Model file for the job. Use its own axes, mm. A direction names the side the tool comes from. Coordinates: 2 decimals unless noted, no trailing zeros. Loops run counter-clockwise (first coordinate to the right, second up) from the corner with the lowest first, then second, coordinate; pieces in that order, holes last.
from build123d import *

# Parameters (mm, degrees)
SZKIC1_R                    = 37.5
SZKIC1_R_2                  = 22.5
DODANIE_WYCI_GNI_CIE1_DEPTH = 41
SZKIC2_R                    = 35
SZKIC2_R_2                  = 25
WYTNIJ_WYCI_GNI_CIE1_DEPTH  = 1
SZKIC3_R                    = 5.05
SZKIC3_R_2                  = 37.5
DODANIE_WYCI_GNI_CIE2_DEPTH = 10
SZYK_KO_OWY1_OUTLINE_R      = 5.05
SZYK_KO_OWY1_DEPTH          = 10


# Read off the part's stored shape, not the designer's step: Szyk kołowy1
with BuildPart() as part:
    # Szkic1 → Dodanie-wyciągnięcie1 (new body)
    with BuildSketch(Plane.XY):
        Circle(SZKIC1_R)
        Circle(SZKIC1_R_2, mode=Mode.SUBTRACT)
    extrude(amount=DODANIE_WYCI_GNI_CIE1_DEPTH)

    # Szkic2 → Wytnij-wyciągnięcie1 (cut)
    with BuildSketch(Plane.XY.offset(41)):
        Circle(SZKIC2_R)
        Circle(SZKIC2_R_2, mode=Mode.SUBTRACT)
    wytnij_wyci_gni_cie1 = extrude(amount=-WYTNIJ_WYCI_GNI_CIE1_DEPTH, mode=Mode.SUBTRACT)

    # Lustro1: Wytnij-wyciągnięcie1 across plane
    add(wytnij_wyci_gni_cie1.mirror(Plane.XY.offset(20.5)), mode=Mode.SUBTRACT)

    # Szkic3 → Dodanie-wyciągnięcie2 (add)
    with BuildSketch(Plane.XY):
        with BuildLine():
            ThreePointArc((-27.971489431, -55.891374818), (44.194173824, 44.194173824), (-55.891374818, -27.971489431))
            ThreePointArc((-55.891374818, -27.971489431), (-30.0520382, -30.0520382), (-27.971489431, -55.891374818))
        make_face()
        with Locations((0, -53)):
            Circle(SZKIC3_R, mode=Mode.SUBTRACT)
        Circle(SZKIC3_R_2, mode=Mode.SUBTRACT)
    extrude(amount=DODANIE_WYCI_GNI_CIE2_DEPTH)

    # Szyk kołowy1 outline → Szyk kołowy1 (cut)
    with BuildSketch(Plane.XY):
        with Locations((-53, 0)):
            Circle(SZYK_KO_OWY1_OUTLINE_R)
        with BuildLine():
            ThreePointArc((-55.891374818, 27.971489431), (-30.0520382, 30.0520382), (-27.971489431, 55.891374818))
            ThreePointArc((-27.971489431, 55.891374818), (-44.194173824, 44.194173824), (-55.891374818, 27.971489431))
        make_face()
        with BuildLine():
            ThreePointArc((27.971489431, -55.891374818), (44.194173824, -44.194173824), (55.891374818, -27.971489431))
            ThreePointArc((55.891374818, -27.971489431), (30.0520382, -30.0520382), (27.971489431, -55.891374818))
        make_face()
        with BuildLine():
            ThreePointArc((55.891374818, 27.971489431), (44.194173824, 44.194173824), (27.971489431, 55.891374818))
            ThreePointArc((27.971489431, 55.891374818), (30.0520382, 30.0520382), (55.891374818, 27.971489431))
        make_face()
        with Locations((0, 53)):
            Circle(SZYK_KO_OWY1_OUTLINE_R)
        with Locations((53, 0)):
            Circle(SZYK_KO_OWY1_OUTLINE_R)
    extrude(amount=SZYK_KO_OWY1_DEPTH, mode=Mode.SUBTRACT)


solid = part.part
Q1. Which spindle directions (+Z, -Z, +X, -X, +Y, -Y) get a long thin tool onto all of the face, cutting with end or side? Do faces 4 (the flat face through (-22.34, 3.82, 41)), 5 (the cylindrical face through (-27.77, -21.3, 40.51)), 6 (the flat face through (-24, 8, 1)). Say none if no direction does.
Answers:
face 4: +Z, +X, -X, +Y, -Y
face 5: +Z
face 6: -Z
Q2. Slice it at A-A (x = 19). List the corners of the cut face in (y, z), and give its area (3 significant figures).
Answers:
outline: (-59.54, 0) - (-29.39, 0) - (-29.39, 1) - (-16.25, 1) - (-16.25, 0) - (-12.05, 0) - (-12.05, 41) - (-16.25, 41) - (-16.25, 40) - (-29.39, 40) - (-29.39, 41) - (-32.33, 41) - (-32.33, 10) - (-59.54, 10) - close; (12.05, 0) - (16.25, 0) - (16.25, 1) - (29.39, 1) - (29.39, 0) - (59.54, 0) - (59.54, 10) - (32.33, 10) - (32.33, 41) - (29.39, 41) - (29.39, 40) - (16.25, 40) - (16.25, 41) - (12.05, 41) - close
area: 2,150 mm2
Q3. Drill centre lines: line 1 (Y direction, x = 0, z = 2); line 2 (Y direction, x = 0, z = 0.35); line 3 (Z direction, x = 19, y = 53.5). Where is each one in solid material? Low to high.
Answers:
line 1: y = -62.5 to -58.05, -47.95 to -22.5, 22.5 to 47.95, 58.05 to 62.5
line 2: y = -62.5 to -58.05, -47.95 to -35, -25 to -22.5, 22.5 to 25, 35 to 47.95, 58.05 to 62.5
line 3: z = 0 to 10
Q4. Slice it at C-C (y = 21). List the corners of the cut face in (x, z), and give its area (3 significant figures).
Answers:
outline: (-58.87, 0) - (-28, 0) - (-28, 1) - (-13.56, 1) - (-13.56, 0) - (-8.08, 0) - (-8.08, 41) - (-13.56, 41) - (-13.56, 40) - (-28, 40) - (-28, 41) - (-31.07, 41) - (-31.07, 10) - (-58.87, 10) - close; (8.08, 0) - (13.56, 0) - (13.56, 1) - (28, 1) - (28, 0) - (58.87, 0) - (58.87, 10) - (31.07, 10) - (31.07, 41) - (28, 41) - (28, 40) - (13.56, 40) - (13.56, 41) - (8.08, 41) - close
area: 2,380 mm2
Q5. Slice it at D-D (x = 0). Count the separate pieces of the cut face and the enclosed holes in it, and give its area (3 significant figures).
Answers:
separate pieces: 4
enclosed holes: 0
area: 1,490 mm2
Q6. Slice it at B-B (z = 5). List the corners of the cut face in (x, y), and give its area (3 significant figures).
Answers:
outline: (-55.89, -27.97) arc R20 cw to (-27.97, -55.89) arc R62.5 ccw to (27.97, -55.89) arc R20 cw to (55.89, -27.97) arc R62.5 ccw to (55.89, 27.97) arc R20 cw to (27.97, 55.89) arc R62.5 ccw to (-27.97, 55.89) arc R20 cw to (-55.89, 27.97) arc R62.5 ccw to start; hole circle Ø10.1 at (-53, 0); hole circle Ø45 at (0, 0); hole circle Ø10.1 at (0, -53); hole circle Ø10.1 at (0, 53); hole circle Ø10.1 at (53, 0)
area: 8,020 mm2
Q7. Flat gauge pins, fed straight in: P1, Ø12, axis at y = 9, z = 25, coming from the -X side; P2, Ø13, axis at x = 53, y = 0, coming from the +Z side; P3, Ø4, axis at y = -20.5, z = 31.5, coming from the -X side. Where does each tip first touch, or does it go through?
Answers:
P1: stops at x = -37.38
P2: stops at z = 10
P3: stops at x = -32.62
Q8. Mould opens along X. For faces 1 (the cylindrical face through (-62.5, 0.4, 4.9)), 2 (the flat face through (-31, 17, 41)), 3 (the cylindrical face through (-30.33, -29.78, 4.93)) say: +X half, -X half, draft (parallel to the pull), parting line (faces both ways), or undercut.
Answers:
face 1: -X half
face 2: draft
face 3: undercut
